Can you work these out from the model? Positions are in its coordinate system, mm. A direction names the side the tool comes from. Coordinates: 2 decimals unless noted, no trailing zeros. Order: outer loops, then holes, each group sorted by start corner. A loop starts at its lowest first (then second) coordinate and runs counter-clockwise, first axis right, second up. Notation, with made-up numbers: (47.5, 82) -> (86.5, 82) arc R19 ccw to (86.5, 95) -> close; hole circle Ø9 at (59.25, -25). An arc over 180 degrees is marked (long way). Return JSON: item names as keys, results as strings. Group by question number.
1) If we section it at A-A, the plane y = 56.5: Please give me the cut outline in (x, z), then the cut area to 3 significant figures.
2) If we section it at D-D, the plane x = 10: Please give me the cut outline in (y, z), then the cut area to 3 significant figures.
3) If we section it at C-C, the plane z = -4: Please give me the cut outline in (x, y), then the cut area to 3 significant figures.
4) If we section it at B-B, the plane x = 25: Please give me the cut outline in (y, z), then the cut area to 3 significant figures.
5) For faces 1 (the cylindrical face through (34.54, 78.52, -3)), 2 (the flat face through (47, 36, 0)), which set-ups out of +Z, -Z, +X, -X, +Y, -Y let a thin tool reach every point of the face, with its end or its side?
6) For pin 1 (12 mm diameter, centred on y = 45.5, z = -10.5, fed in from -X); pin 2 (19 mm diameter, centred on x = 23.5, z = 2, fed in from -Y), each with a flat end and sliding along its axis, tell me the tip position at first contact or that it passes through.
7) Thinking about a two-plate mould opening in Y: for faces 3 (the cylindrical face through (3.9, 76.14, 0.28)), 4 (the cylindrical face through (1.48, 15.12, -1.08)), 5 (the flat face through (0, 38, 0)), which applies, +Y half, -Y half, draft (parallel to the pull), parting line (faces both ways), or undercut?
8) If I drill on probe 1 along X at (y, z) = (53.5, -8); probe 2 along Z at (x, y) = (25, 79.15); probe 3 along Y at (x, z) = (48.65, 0), over which ranges is the centre line in solid material (lowest first)? Write a range as from..to.
Autodesk Inventor part; units mm, degrees
ref_plane "YZ Plane" through (0, 0, 0) normal (1, 0, 0) x (0, 1, 0)
ref_plane "XZ Plane" through (0, 0, 0) normal (0, 1, 0) x (-1, 0, 0)
ref_plane "XY Plane" through (0, 0, 0) normal (0, 0, 1) x (1, 0, 0)
sketch "Esboço1" plane through (0, 0, 0) normal (0, 0, 1) x (1, 0, 0)
  line L0 (0, 0) -> (0, 80)
  line L1 (0, 80) -> (50, 80)
  line L2 (50, 80) -> (50, 0)
  line L3 (47, 0) -> (47, 77)
  line L4 (47, 77) -> (3, 77)
  line L5 (3, 77) -> (3, 0)
  line L6 (0, 0) -> (3, 0)
  line L7 (47, 0) -> (50, 0)
  dimension "d0" = 80
  dimension "d1" = 3
  dimension "d2" = 3
  dimension "d3" = 50
  dimension "d4" = 3
extrude "Extrusão1" add sketch "Esboço1" along normal mid plane 40
fillet "Arredondamento1" radius 20 1 edges at (48.5, 0, 20)
fillet "Arredondamento2" radius 20 1 edges at (48.5, 0, -20)
fillet "Arredondamento3" radius 20 1 edges at (1.5, 0, -20)
fillet "Arredondamento4" radius 20 1 edges at (1.5, 0, 20)
fillet "Arredondamento5" radius 3 1 edges at (50, 80, 0)
fillet "Arredondamento6" radius 3 1 edges at (0, 80, 0)
fillet "Arredondamento7" radius 3 1 edges at (3, 77, 0)
fillet "Arredondamento8" radius 3 1 edges at (47, 77, 0)
sketch "Esboço2" plane through (0, 20, 0) normal (-1, 0, 0) x (0, 0, 1)
  circle A0 centre (0, 0) radius 5
  line L0 (20, 60) -> (-20, 60)
  point P0 (0, -20)
  dimension "d15" = 10
  dimension "d16" = 60
extrude "Extrusão2" cut sketch "Esboço2" against normal blind 50
sketch "Esboço3" plane through (47, 80, 20) normal (0, 1, 0) x (1, 0, 0)
  line L0 (-44, 25) -> (-44, 15)
  line L1 (-44, 20) -> (0, 20)
  line L2 (0, 40) -> (0, 0)
  circle A0 centre (-22, 20) radius 10
  point P0 (-47, 20)
  dimension "d19" = 20
extrude "Extrusão3" cut sketch "Esboço3" against normal blind 50
properties part number "suporte"
Result sheet:
{
 "1": {"outline": "(0, -20) -> (3, -20) -> (3, 20) -> (0, 20) -> close; (47, -20) -> (50, -20) -> (50, 20) -> (47, 20) -> close", "area": "240 mm2"},
 "2": {"outline": "(77, -20) -> (80, -20) -> (80, 20) -> (77, 20) -> close", "area": "120 mm2"},
 "3": {"outline": "(0, 0.4) -> (3, 0.4) -> (3, 17) -> (0, 17) -> close; (0, 23) -> (3, 23) -> (3, 74) arc R3 cw to (6, 77) -> (15.83, 77) -> (15.83, 80) -> (3, 80) arc R3 ccw to (0, 77) -> close; (34.17, 77) -> (44, 77) arc R3 cw to (47, 74) -> (47, 23) -> (50, 23) -> (50, 77) arc R3 ccw to (47, 80) -> (34.17, 80) -> close; (47, 0.4) -> (50, 0.4) -> (50, 17) -> (47, 17) -> close", "area": "519 mm2"},
 "4": {"outline": "(77, -20) -> (80, -20) -> (80, -10) -> (77, -10) -> close; (77, 10) -> (80, 10) -> (80, 20) -> (77, 20) -> close", "area": "60.0 mm2"},
 "5": {"face 1": "+Y, -Y", "face 2": "+Z, -Z, -Y"},
 "6": {"pin 1": "stops at x = 0", "pin 2": "stops at y = 77"},
 "7": {"face 3": "-Y half", "face 4": "undercut", "face 5": "draft"},
 "8": {"probe 1": "x = 0..3, 47..50", "probe 2": "z = -20..-10, 10..20", "probe 3": "y = 0..15, 25..79.51"}
}
